from build123d import *

# Parameters (mm, degrees)
SKETCH_1_R          = 2.75
SKETCH_1_R_2        = 1.6
EXTRUDE_1_DEPTH     = 5
EXTRUDE_START       = -1.5
SKETCH_2_R          = 2.75
SKETCH_2_R_2        = 1.6
EXTRUDE_2_DEPTH     = 1.5
SKETCH_3_W          = 127
SKETCH_3_H          = 8
CUT_EXTRUDE_1_DEPTH = 2
CHAMFER_1_SIZE2     = 2
CHAMFER_1_SIZE      = 10


with BuildPart() as part:
    # 草圖1 → 填料-伸長1 (new body)
    with BuildSketch(Plane.XY):
        with BuildLine():
            Line((-53.111291809, 4), (80.888708191, 4))
            ThreePointArc((80.888708191, 4), (84.888708191, 0), (80.888708191, -4))
            Line((80.888708191, -4), (-53.111291809, -4))
            ThreePointArc((-53.111291809, -4), (-57.111291809, 0), (-53.111291809, 4))
        make_face()
        with Locations((80.888708191, 0)):
            Circle(SKETCH_1_R, mode=Mode.SUBTRACT)
        with Locations((-53.111291809, 0)):
            Circle(SKETCH_1_R_2, mode=Mode.SUBTRACT)
        with Locations((13.888708191, 0)):
            Circle(SKETCH_1_R_2, mode=Mode.SUBTRACT)
    extrude(amount=EXTRUDE_1_DEPTH)

    # 草圖2 → 填料-伸長2 (add)
    with BuildSketch(Plane.XY.offset(5).offset(EXTRUDE_START)):
        with Locations((80.888708191, 0)):
            Circle(SKETCH_2_R)
        with Locations((80.888708191, 0)):
            Circle(SKETCH_2_R_2, mode=Mode.SUBTRACT)
    extrude(amount=EXTRUDE_2_DEPTH)

    # 草圖3 → 除料-伸長1 (cut)
    with BuildSketch(Plane.XY.offset(5)):
        with Locations((2.388708191, 0)):
            Rectangle(SKETCH_3_W, SKETCH_3_H)
    extrude(amount=-CUT_EXTRUDE_1_DEPTH, mode=Mode.SUBTRACT)

    # 導角1
    chamfer_1_edges = [part.edges().sort_by_distance(p)[0] for p in [
        (65.888708191, 0, 5),
    ]]
    chamfer_1_side = [part.faces().sort_by_distance(p)[0] for p in [
        (65.928708191, 0, 5),
    ]]
    chamfer(chamfer_1_edges, length=CHAMFER_1_SIZE - 0.0001, length2=CHAMFER_1_SIZE2 - 0.0001, reference=chamfer_1_side[0])  # a hair under: the kernel refuses the full size


solid = part.part
Work out the finished part from the listing and answer in its coordinate system (mm). A direction names the side the tool comes from. Give positions to 0.01 mm unless a question says otherwise; leave off trailing zeros. Write each loop counter-clockwise with the first axis right and the second up, starting at its lowest first coordinate (ties: lowest second). Pieces come first, ordered by that corner, then holes. Notation, with made-up numbers: M -3,-35 L 5,-35 A27 cw 5,-16 Z; hole C 29,-37.5 d11. An arc over 180 degrees is marked long. Answer as CSV lines item,"result".
Q1. A tool of negligible diameter and unlimited length cuts with its end or side. For faces 4 (the flat face through (4, 0, 3)), 5 (the flat face through (81, -2, 3.5)), 6 (the cylindrical face through (84.888, 0.088, 2.465)), from which of +Z, -Z, +X, -X, +Y, -Y can it reach the whole face along a straight path? Write none if from no direction.
A:
face 4,"+Z, -X, +Y, -Y"
face 5,"-Z"
face 6,"+Z, -Z, +X"
Q2. A cutting plane is placed at B-B on x = -36. Write down the section's boundary in (y, z).
A:
outline,"M -4,0 L 4,0 L 4,3 L -4,3 Z"
Q3. The mould has two halves that part along Y. Classify faces 1 (the flat face through (15, -4, 1)), 2 (the cylindrical face through (78.14, 0.12, 1.73)), 3 (the flat face through (15, 2, 0)): +Y half, -Y half, draft (parallel to the pull), parting line (faces both ways), or undercut.
A:
face 1,"-Y half"
face 2,"undercut"
face 3,"draft"
Q4. Given P1, Ø2.5, axis at x = -53.11, y = 0, coming from the -Z side; P2, Ø1, axis at y = -1, z = 1, coming from the +X side; P3, Ø4, axis at x = 13.89, y = 0, coming from the +Z side; P4, Ø4.5, axis at x = 80.89, y = 0, coming from the -Z side, each flat-ended and moving along its own axis, determine where each tip first touches the part or whether it passes through.
A:
P1,"passes through"
P2,"stops at x = 84.86"
P3,"stops at z = 3"
P4,"stops at z = 3.5"
Q5. Find the intervals of material crossed by probe 1 along Z at (x, y) = (-33.5, 0); probe 2 along X at (y, z) = (2.25, 2.05); probe 3 along X at (y, z) = (3, 0.55), in increasing order. Write a range as [from, to].
A:
probe 1,"z = [0, 3]"
probe 2,"x = [-56.42, 79.31], [82.47, 84.2]"
probe 3,"x = [-55.76, 83.53]"
Q6. A cutting plane is placed at A-A on y = 0. Count the separate pieces of the cut face and the enclosed holes in it, plus the area to 3 significant figures.
A:
separate pieces,"4"
enclosed holes,"0"
area,"411 mm²"
